```python
from build123d import *

# Parameters (mm, degrees)
SKETCH1_R           = 1.75
SKETCH1_R_2         = 1
BOSS_EXTRUDE1_DEPTH = 5
SKETCH2_R           = 3.14
SKETCH2_R_2         = 1.75
SKETCH2_R_3         = 1
BOSS_EXTRUDE2_DEPTH = 1
SKETCH2_4_R         = 3.14
BOSS_EXTRUDE3_DEPTH = 8
FILLET1_R           = 0.5
FILLET2_R           = 0.2


with BuildPart() as part:
    # Sketch1 → Boss-Extrude1 (new body)
    with BuildSketch(Plane.XY):
        Circle(SKETCH1_R)
        Circle(SKETCH1_R_2, mode=Mode.SUBTRACT)
    extrude(amount=BOSS_EXTRUDE1_DEPTH)

    # Sketch2 → Boss-Extrude2 (add)
    # profile 1 of 12: a face of its own
    with BuildSketch(Plane.XY.offset(5)):
        Circle(SKETCH2_R)
        with BuildLine():
            ThreePointArc((-0.94, -2.25166605), (0, -2.44), (0.94, -2.25166605))
            Line((0.94, -2.25166605), (0.94, -0.94))
            Line((0.94, -0.94), (2.25166605, -0.94))
            ThreePointArc((2.25166605, -0.94), (2.44, 0), (2.25166605, 0.94))
            Line((2.25166605, 0.94), (0.94, 0.94))
            Line((0.94, 0.94), (0.94, 2.25166605))
            ThreePointArc((0.94, 2.25166605), (0, 2.44), (-0.94, 2.25166605))
            Line((-0.94, 2.25166605), (-0.94, 0.94))
            Line((-0.94, 0.94), (-2.25166605, 0.94))
            ThreePointArc((-2.25166605, 0.94), (-2.44, 0), (-2.25166605, -0.94))
            Line((-2.25166605, -0.94), (-0.94, -0.94))
            Line((-0.94, -0.94), (-0.94, -2.25166605))
        make_face(mode=Mode.SUBTRACT)
    # profile 2 of 12: a face of its own
    with BuildSketch(Plane.XY.offset(5)):
        Circle(SKETCH2_R_2)
    # profile 3 of 12: a face of its own
    with BuildSketch(Plane.XY.offset(5)):
        with BuildLine():
            Line((-0.94, 0.94), (-0.94, 1.476109752))
            ThreePointArc((-0.94, 1.476109752), (-1.237436867, 1.237436867), (-1.476109752, 0.94))
            Line((-1.476109752, 0.94), (-0.94, 0.94))
        make_face()
    # profile 4 of 12: a face of its own
    with BuildSketch(Plane.XY.offset(5)):
        with BuildLine():
            ThreePointArc((-1.476109752, -0.94), (-1.75, 0), (-1.476109752, 0.94))
            Line((-1.476109752, 0.94), (-2.25166605, 0.94))
            ThreePointArc((-2.25166605, 0.94), (-2.44, 0), (-2.25166605, -0.94))
            Line((-2.25166605, -0.94), (-1.476109752, -0.94))
        make_face()
    # profile 5 of 12: a face of its own
    with BuildSketch(Plane.XY.offset(5)):
        with BuildLine():
            Line((1.476109752, 0.94), (0.94, 0.94))
            Line((0.94, 0.94), (0.94, 1.476109752))
            ThreePointArc((0.94, 1.476109752), (0, 1.75), (-0.94, 1.476109752))
            Line((-0.94, 1.476109752), (-0.94, 0.94))
            Line((-0.94, 0.94), (-1.476109752, 0.94))
            ThreePointArc((-1.476109752, 0.94), (-1.75, 0), (-1.476109752, -0.94))
            Line((-1.476109752, -0.94), (-0.94, -0.94))
            Line((-0.94, -0.94), (-0.94, -1.476109752))
            ThreePointArc((-0.94, -1.476109752), (0, -1.75), (0.94, -1.476109752))
            Line((0.94, -1.476109752), (0.94, -0.94))
            Line((0.94, -0.94), (1.476109752, -0.94))
            ThreePointArc((1.476109752, -0.94), (1.680132743, -0.489544653), (1.75, 0))
            ThreePointArc((1.75, 0), (1.680132743, 0.489544653), (1.476109752, 0.94))
        make_face()
        Circle(SKETCH2_R_3, mode=Mode.SUBTRACT)
    # profile 6 of 12: a face of its own
    with BuildSketch(Plane.XY.offset(5)):
        Circle(SKETCH2_R_3)
    # profile 7 of 12: a face of its own
    with BuildSketch(Plane.XY.offset(5)):
        with BuildLine():
            ThreePointArc((-0.94, 1.476109752), (0, 1.75), (0.94, 1.476109752))
            Line((0.94, 1.476109752), (0.94, 2.25166605))
            ThreePointArc((0.94, 2.25166605), (0, 2.44), (-0.94, 2.25166605))
            Line((-0.94, 2.25166605), (-0.94, 1.476109752))
        make_face()
    # profile 8 of 12: a face of its own
    with BuildSketch(Plane.XY.offset(5)):
        with BuildLine():
            Line((0.94, 1.476109752), (0.94, 0.94))
            Line((0.94, 0.94), (1.476109752, 0.94))
            ThreePointArc((1.476109752, 0.94), (1.237436867, 1.237436867), (0.94, 1.476109752))
        make_face()
    # profile 9 of 12: a face of its own
    with BuildSketch(Plane.XY.offset(5)):
        with BuildLine():
            Line((2.25166605, 0.94), (1.476109752, 0.94))
            ThreePointArc((1.476109752, 0.94), (1.680132743, 0.489544653), (1.75, 0))
            ThreePointArc((1.75, 0), (1.680132743, -0.489544653), (1.476109752, -0.94))
            Line((1.476109752, -0.94), (2.25166605, -0.94))
            ThreePointArc((2.25166605, -0.94), (2.44, 0), (2.25166605, 0.94))
        make_face()
    # profile 10 of 12: a face of its own
    with BuildSketch(Plane.XY.offset(5)):
        with BuildLine():
            ThreePointArc((0.94, -1.476109752), (1.237436867, -1.237436867), (1.476109752, -0.94))
            Line((1.476109752, -0.94), (0.94, -0.94))
            Line((0.94, -0.94), (0.94, -1.476109752))
        make_face()
    # profile 11 of 12: a face of its own
    with BuildSketch(Plane.XY.offset(5)):
        with BuildLine():
            Line((0.94, -2.25166605), (0.94, -1.476109752))
            ThreePointArc((0.94, -1.476109752), (0, -1.75), (-0.94, -1.476109752))
            Line((-0.94, -1.476109752), (-0.94, -2.25166605))
            ThreePointArc((-0.94, -2.25166605), (0, -2.44), (0.94, -2.25166605))
        make_face()
    # profile 12 of 12: a face of its own
    with BuildSketch(Plane.XY.offset(5)):
        with BuildLine():
            Line((-0.94, -0.94), (-1.476109752, -0.94))
            ThreePointArc((-1.476109752, -0.94), (-1.237436867, -1.237436867), (-0.94, -1.476109752))
            Line((-0.94, -1.476109752), (-0.94, -0.94))
        make_face()
    extrude(amount=BOSS_EXTRUDE2_DEPTH)

    # Sketch2_4 → Boss-Extrude3 (add)
    with BuildSketch(Plane.XY.offset(5)):
        Circle(SKETCH2_4_R)
        with BuildLine():
            Line((0.94, 0.94), (2.25166605, 0.94))
            ThreePointArc((2.25166605, 0.94), (2.44, 0), (2.25166605, -0.94))
            Line((2.25166605, -0.94), (0.94, -0.94))
            Line((0.94, -0.94), (0.94, -2.25166605))
            ThreePointArc((0.94, -2.25166605), (0, -2.44), (-0.94, -2.25166605))
            Line((-0.94, -2.25166605), (-0.94, -0.94))
            Line((-0.94, -0.94), (-2.25166605, -0.94))
            ThreePointArc((-2.25166605, -0.94), (-2.44, 0), (-2.25166605, 0.94))
            Line((-2.25166605, 0.94), (-0.94, 0.94))
            Line((-0.94, 0.94), (-0.94, 2.25166605))
            ThreePointArc((-0.94, 2.25166605), (0, 2.44), (0.94, 2.25166605))
            Line((0.94, 2.25166605), (0.94, 0.94))
        make_face(mode=Mode.SUBTRACT)
    extrude(amount=BOSS_EXTRUDE3_DEPTH)

    # Fillet1
    fillet1_edges = [part.edges().sort_by_distance(p)[0] for p in [
        (-3.14, 0, 5),
        (-1.75, 0, 5),
    ]]
    fillet(fillet1_edges, radius=FILLET1_R)

    # Fillet2
    fillet2_edges = [part.edges().sort_by_distance(p)[0] for p in [
        (-0.94, -0.94, 9.5),
        (-0.94, 0.94, 9.5),
        (0.94, 0.94, 9.5),
        (0.94, -0.94, 9.5),
    ]]
    fillet(fillet2_edges, radius=FILLET2_R)


solid = part.part
```
Geometry check sheet. Reference: the model listing, model coordinates, mm. A direction names the side the tool comes from. Coordinates: 2 decimals unless noted, no trailing zeros. Order: outer loops, then holes, each group sorted by start corner. A loop starts at its lowest first (then second) coordinate and runs counter-clockwise, first axis right, second up. Notation, with made-up numbers: (54.25, 18) - (59.25, 18) arc R27 ccw to (59.25, 34) - close; hole circle Ø8 at (41.25, 44). An arc over 180 degrees is marked (long way). Answer in a Markdown table with one row per item. Add a question column.
1. Section check A-A (x = 0). Enter the section's corners in (y, z).
2. Material ranges on L1, parallel to Y at x = 0, z = 2.2; L2, parallel to Z at x = -0.5, y = -0.5; L3, parallel to Z at x = 1, y = 0.25, recorded low to high. Write a range as [from, to].
3. Gauge pin test, flat ends, axial feed: pin 1 Ø1.6 at (x, y) = (0, 0) entering from -Z; pin 2 Ø1.5 at (x, z) = (2.5, 9.5) entering from -Y; pin 3 Ø1.2 at (y, z) = (1.5, 10) entering from -X. Record the tip position at first contact, or that the pin passes through.
4. Section check C-C (z = 4.25). Enter the section's corners in (x, y), plus the area to 3 significant figures.
5. Access from +Z, -Z, +X, -X, +Y, -Y to the whole of each face (thin tool, end or side, straight path). Record for faces 4 (the face through (0.94, 2, 9)), 5 (the face through (0, -1, 2)), 6 (the face through (1.4, -1.4, 13)).
6. Draft check along Y on faces 1 (the face through (1, -1, 0)), 2 (the face through (1.617, -0.67, 2.218)), 3 (the face through (2.44, 0.01, 9.45)). Enter one of: +Y half, -Y half, draft (parallel to the pull), parting line (faces both ways), or undercut.
Data:
| question | item | result |
|---|---|---|
| 1 | outline | (-3.14, 5.5) arc R0.5 ccw to (-2.64, 5) - (-2.25, 5) arc R0.5 cw to (-1.75, 4.5) - (-1.75, 0) - (-1, 0) - (-1, 5) - (1, 5) - (1, 0) - (1.75, 0) - (1.75, 4.5) arc R0.5 cw to (2.25, 5) - (2.64, 5) arc R0.5 ccw to (3.14, 5.5) - (3.14, 13) - (2.44, 13) - (2.44, 6) - (-2.44, 6) - (-2.44, 13) - (-3.14, 13) - close |
| 2 | L1 | y = [-1.75, -1], [1, 1.75] |
| 2 | L2 | z = [5, 6] |
| 2 | L3 | z = [0, 6] |
| 3 | pin 1 | stops at z = 5 |
| 3 | pin 2 | stops at y = -2.61 |
| 3 | pin 3 | stops at x = -3.01 |
| 4 | outline | circle Ø3.5 at (0, 0); hole circle Ø2 at (0, 0) |
| 4 | area | 6.48 mm² |
| 5 | face 4 | +Z |
| 5 | face 5 | -Z |
| 5 | face 6 | +Z, +X, -X, +Y, -Y |
| 6 | face 1 | draft |
| 6 | face 2 | parting line |
| 6 | face 3 | undercut |
